Work out the finished part from the listing and answer in its coordinate system (mm). A direction names the side the tool comes from. Round coordinates to 2 decimals unless told otherwise and drop trailing zeros. Order: outer loops, then holes, each group sorted by start corner. A loop starts at its lowest first (then second) coordinate and runs counter-clockwise, first axis right, second up. Notation, with made-up numbers: (-33, -17) -> (21, -17) arc R20 cw to (21, 16) -> close; hole circle Ø3 at (-25, 83). An arc over 180 degrees is marked (long way). Use a Markdown table: item, result. Add a question column.
Item 1: For a pull along Z with two mould halves and no side action, classify faces 6 (the flat face through (90, 1, 0)), 7 (the flat face through (30.5, 5, 140)), 8 (the cylindrical face through (28.52, 3.48, 97.92)) as +Z half, -Z half, draft (parallel to the pull), parting line (faces both ways), or undercut.
Item 2: Flat-ended cylindrical pins translate along their axes: P1, Ø1, axis at x = 93, z = 76, coming from the -Y side; P2, Ø4, axis at x = 67.5, z = 99.5, coming from the +Y side; P3, Ø3, axis at x = 133, y = 5.5, coming from the +Z side. Find the tip coordinate at first contact, or state that the pin passes through.
Item 3: A cutting plane is placed at B-B, the plane z = 29. Determine the outline of the cut face in (x, y), plus the area to 3 significant figures.
Item 4: A cutting plane is placed at C-C, the plane y = -8. Determine the outline of the cut face in (x, z).
Item 5: A tool of negligible diameter and unlimited length cuts with its end or side. For faces 1 (the flat face through (71, 5, 13)), 2 (the flat face through (131, 7, 13)), 3 (the flat face through (144, 5, 90)), 4 (the flat face through (132, 5, 140)), 5 (the flat face through (81, 0, 77)), from which of +Z, -Z, +X, -X, +Y, -Y can it reach the whole face along a straight path? Write none if from no direction.
Item 6: Find the intervals of material crossed by L1, parallel to X at y = -2, z = 149; L2, parallel to Y at x = 5.5, z = 114.5; L3, parallel to Y at x = 178.5, z = 110.5, in increasing order. Write a range as [from, to].
Item 7: A cutting plane is placed at A-A, the plane z = 77.85. Determine the outline of the cut face in (x, y).
from build123d import *

# Parameters (mm, degrees)
LINEAR_AUSTRAGEN_D_NN1_DEPTH     = 155.5
SKIZZE7_R                        = 2.5
AUFSATZ_LINEAR_AUSTRAGEN3_DEPTH  = 5
SKIZZE8_R                        = 1.5
SCHNITT_LINEAR_AUSTRAGEN1_DEPTH  = 8
SKIZZE12_R                       = 1.5
SCHNITT_LINEAR_AUSTRAGEN4_DEPTH  = 8
SKIZZE13_R                       = 2.5
AUFSATZ_LINEAR_AUSTRAGEN5_DEPTH  = 5
SKIZZE16_R                       = 1.5
SCHNITT_LINEAR_AUSTRAGEN9_DEPTH  = 8
SKIZZE17_R                       = 1.5
SCHNITT_LINEAR_AUSTRAGEN10_DEPTH = 8
SKIZZE18_R                       = 2.5
AUFSATZ_LINEAR_AUSTRAGEN6_DEPTH  = 5
SKIZZE21_R                       = 1.5
SCHNITT_LINEAR_AUSTRAGEN13_DEPTH = 8
SKIZZE22_R                       = 1.5
SCHNITT_LINEAR_AUSTRAGEN14_DEPTH = 8
SKIZZE20_R                       = 1.2
AUFSATZ_LINEAR_AUSTRAGEN7_DEPTH  = 5
SKIZZE19_R                       = 1.2
AUFSATZ_LINEAR_AUSTRAGEN8_DEPTH  = 5
SKIZZE15_R                       = 1.2
AUFSATZ_LINEAR_AUSTRAGEN9_DEPTH  = 5
SKIZZE14_R                       = 1.2
AUFSATZ_LINEAR_AUSTRAGEN11_DEPTH = 5
SKIZZE10_R                       = 1.2
AUFSATZ_LINEAR_AUSTRAGEN12_DEPTH = 5
SKIZZE11_R                       = 1.2
AUFSATZ_LINEAR_AUSTRAGEN13_DEPTH = 5
CUT_EXTRUDE2_DEPTH               = 156.5
SKIZZE23_R                       = 13
SCHNITT_LINEAR_AUSTRAGEN15_DEPTH = 13
SKETCH5_W                        = 1
SKETCH5_H                        = 155.5
CUT_EXTRUDE_THIN1_DEPTH          = 1
SKETCH6_R                        = 2.5
SKETCH6_R_2                      = 1.5
BOSS_EXTRUDE1_DEPTH              = 5
CUT_EXTRUDE3_START               = -2
SKETCH7_R                        = 1.5
CUT_EXTRUDE3_DEPTH               = 2


with BuildPart() as part:
    # Skizze5 → Linear-Austragen-Dünn1 (new body)
    with BuildSketch(Plane.XY):
        with BuildLine():
            Line((-17.5, -12.340428851), (0, -12.340428851))
            Line((0, -12.340428851), (0, 0))
            Line((0, 0), (158.213118455, 0))
            Line((158.213118455, 0), (163.626964647, 0))
            ThreePointArc((163.626964647, 0), (171.029319744, 7.247508118), (181.129906705, 9.549545901))
            ThreePointArc((181.129906705, 9.549545901), (191.077251396, 6.131307404), (197.694328428, -2.044774322))
            Line((197.694328428, -2.044774322), (199.194328428, -2.044774322))
            Line((199.194328428, -2.044774322), (199.194328428, -0.044774322))
            Line((199.194328428, -0.044774322), (198.972575208, -0.044774322))
            ThreePointArc((198.972575208, -0.044774322), (191.667573532, 8.146277022), (181.232439294, 11.546915938))
            ThreePointArc((181.232439294, 11.546915938), (170.592452046, 9.278075868), (162.50625544, 2))
            Line((162.50625544, 2), (158.213118455, 2))
            Line((158.213118455, 2), (-2, 2))
            Line((-2, 2), (-2, -10.340428851))
            Line((-2, -10.340428851), (-17.5, -10.340428851))
            Line((-17.5, -10.340428851), (-17.5, -12.340428851))
        make_face()
    extrude(amount=LINEAR_AUSTRAGEN_D_NN1_DEPTH)

    # Skizze7 → Aufsatz-Linear austragen3 (add)
    with BuildSketch(Plane(origin=(0.013003032, 0, 0), x_dir=(1, 0, 0), z_dir=(0, 1, 0))):
        with Locations((11.5, -11.5)):
            Circle(SKIZZE7_R)
        with Locations((69.5, -11.5)):
            Circle(SKIZZE7_R)
        with Locations((11.5, -60.5)):
            Circle(SKIZZE7_R)
        with Locations((69.5, -60.5)):
            Circle(SKIZZE7_R)
    extrude(amount=AUFSATZ_LINEAR_AUSTRAGEN3_DEPTH)

    # Skizze8 → Schnitt-Linear austragen1 (cut)
    with BuildSketch(Plane(origin=(0, 5, 0), x_dir=(1, 0, 0), z_dir=(0, 1, 0))):
        with Locations((11.513003032, -11.5)):
            Circle(SKIZZE8_R)
    extrude(amount=-SCHNITT_LINEAR_AUSTRAGEN1_DEPTH, mode=Mode.SUBTRACT)

    # Skizze12 → Schnitt-Linear austragen4 (cut)
    with BuildSketch(Plane(origin=(0, 5, 0), x_dir=(1, 0, 0), z_dir=(0, 1, 0))):
        with Locations((69.513003032, -11.5)):
            Circle(SKIZZE12_R)
    extrude(amount=-SCHNITT_LINEAR_AUSTRAGEN4_DEPTH, mode=Mode.SUBTRACT)

    # Skizze13 → Aufsatz-Linear austragen5 (add)
    with BuildSketch(Plane(origin=(0.013003032, 0, 0), x_dir=(1, 0, 0), z_dir=(0, 1, 0))):
        with Locations((130, -140)):
            Circle(SKIZZE13_R)
        with Locations((102.1, -140)):
            Circle(SKIZZE13_R)
        with Locations((145.2, -89.2)):
            Circle(SKIZZE13_R)
        with Locations((97.4, -88.1)):
            Circle(SKIZZE13_R)
    extrude(amount=AUFSATZ_LINEAR_AUSTRAGEN5_DEPTH)

    # Skizze16 → Schnitt-Linear austragen9 (cut)
    with BuildSketch(Plane(origin=(0, 5, 0), x_dir=(1, 0, 0), z_dir=(0, 1, 0))):
        with Locations((102.113003032, -140)):
            Circle(SKIZZE16_R)
    extrude(amount=-SCHNITT_LINEAR_AUSTRAGEN9_DEPTH, mode=Mode.SUBTRACT)

    # Skizze17 → Schnitt-Linear austragen10 (cut)
    with BuildSketch(Plane(origin=(0, 5, 0), x_dir=(1, 0, 0), z_dir=(0, 1, 0))):
        with Locations((130.013003032, -140)):
            Circle(SKIZZE17_R)
    extrude(amount=-SCHNITT_LINEAR_AUSTRAGEN10_DEPTH, mode=Mode.SUBTRACT)

    # Skizze18 → Aufsatz-Linear austragen6 (add)
    with BuildSketch(Plane(origin=(0.013003032, 0, 0), x_dir=(1, 0, 0), z_dir=(0, 1, 0))):
        with Locations((68.430981836, -140)):
            Circle(SKIZZE18_R)
        with Locations((28.830981836, -140)):
            Circle(SKIZZE18_R)
        with Locations((28.83098184, -100.4)):
            Circle(SKIZZE18_R)
        with Locations((68.430981836, -100.4)):
            Circle(SKIZZE18_R)
    extrude(amount=AUFSATZ_LINEAR_AUSTRAGEN6_DEPTH)

    # Skizze21 → Schnitt-Linear austragen13 (cut)
    with BuildSketch(Plane(origin=(0, 5, 0), x_dir=(1, 0, 0), z_dir=(0, 1, 0))):
        with Locations((28.843984868, -140)):
            Circle(SKIZZE21_R)
    extrude(amount=-SCHNITT_LINEAR_AUSTRAGEN13_DEPTH, mode=Mode.SUBTRACT)

    # Skizze22 → Schnitt-Linear austragen14 (cut)
    with BuildSketch(Plane(origin=(0, 5, 0), x_dir=(1, 0, 0), z_dir=(0, 1, 0))):
        with Locations((68.443984868, -140)):
            Circle(SKIZZE22_R)
    extrude(amount=-SCHNITT_LINEAR_AUSTRAGEN14_DEPTH, mode=Mode.SUBTRACT)

    # Skizze20 → Aufsatz-Linear austragen7 (add)
    with BuildSketch(Plane(origin=(0, 5, 0), x_dir=(1, 0, 0), z_dir=(0, 1, 0))):
        with Locations((28.843984872, -100.4)):
            Circle(SKIZZE20_R)
    extrude(amount=AUFSATZ_LINEAR_AUSTRAGEN7_DEPTH)

    # Skizze19 → Aufsatz-Linear austragen8 (add)
    with BuildSketch(Plane(origin=(0, 5, 0), x_dir=(1, 0, 0), z_dir=(0, 1, 0))):
        with Locations((68.443984868, -100.4)):
            Circle(SKIZZE19_R)
    extrude(amount=AUFSATZ_LINEAR_AUSTRAGEN8_DEPTH)

    # Skizze15 → Aufsatz-Linear austragen9 (add)
    with BuildSketch(Plane(origin=(0, 5, 0), x_dir=(1, 0, 0), z_dir=(0, 1, 0))):
        with Locations((97.413003032, -88.1)):
            Circle(SKIZZE15_R)
    extrude(amount=AUFSATZ_LINEAR_AUSTRAGEN9_DEPTH)

    # Skizze14 → Aufsatz-Linear austragen11 (add)
    with BuildSketch(Plane(origin=(0, 5, 0), x_dir=(1, 0, 0), z_dir=(0, 1, 0))):
        with Locations((145.213003032, -89.2)):
            Circle(SKIZZE14_R)
    extrude(amount=AUFSATZ_LINEAR_AUSTRAGEN11_DEPTH)

    # Skizze10 → Aufsatz-Linear austragen12 (add)
    with BuildSketch(Plane(origin=(0, 5, 0), x_dir=(1, 0, 0), z_dir=(0, 1, 0))):
        with Locations((11.513003032, -60.5)):
            Circle(SKIZZE10_R)
    extrude(amount=AUFSATZ_LINEAR_AUSTRAGEN12_DEPTH)

    # Skizze11 → Aufsatz-Linear austragen13 (add)
    with BuildSketch(Plane(origin=(0, 5, 0), x_dir=(1, 0, 0), z_dir=(0, 1, 0))):
        with Locations((69.513003032, -60.5)):
            Circle(SKIZZE11_R)
    extrude(amount=AUFSATZ_LINEAR_AUSTRAGEN13_DEPTH)

    # Sketch3 → Cut-Extrude2 (cut, through all)
    with BuildSketch(Plane(origin=(0, 0, 0), x_dir=(-1, 0, 0), z_dir=(0, 0, -1))):
        Polygon((17.5, -10.340428851), (15.5, -12.340428851), (17.5, -12.340428851), align=None)
    extrude(amount=-CUT_EXTRUDE2_DEPTH, mode=Mode.SUBTRACT)

    # Skizze23 → Schnitt-Linear austragen15 (cut)
    with BuildSketch(Plane(origin=(0, 2, 0), x_dir=(1, 0, 0), z_dir=(0, 1, 0))):
        with Locations((181, -77.85)):
            Circle(SKIZZE23_R)
    extrude(amount=SCHNITT_LINEAR_AUSTRAGEN15_DEPTH, mode=Mode.SUBTRACT)

    # Sketch5 → Cut-Extrude-Thin1 (cut)
    with BuildSketch(Plane(origin=(0, 2, 0), x_dir=(1, 0, 0), z_dir=(0, 1, 0))):
        with Locations((80.25312772, -77.75)):
            Rectangle(SKETCH5_W, SKETCH5_H)
    extrude(amount=-CUT_EXTRUDE_THIN1_DEPTH, mode=Mode.SUBTRACT)

    # Sketch6 → Boss-Extrude1 (add)
    with BuildSketch(Plane(origin=(0, 2, 0), x_dir=(1, 0, 0), z_dir=(0, 1, 0))):
        with Locations((130.01300303, -11.5)):
            Circle(SKETCH6_R)
        with Locations((130.01300303, -11.5)):
            Circle(SKETCH6_R_2, mode=Mode.SUBTRACT)
    extrude(amount=BOSS_EXTRUDE1_DEPTH)

    # Sketch7 → Cut-Extrude3 (cut)
    with BuildSketch(Plane(origin=(0, 2, 0), x_dir=(1, 0, 0), z_dir=(0, 1, 0)).offset(CUT_EXTRUDE3_START)):
        with Locations((130.01300303, -11.5)):
            Circle(SKETCH7_R)
    extrude(amount=CUT_EXTRUDE3_DEPTH, mode=Mode.SUBTRACT)


solid = part.part
Reported:
| question | item | result |
|---|---|---|
| 1 | face 6 | -Z half |
| 1 | face 7 | draft |
| 1 | face 8 | undercut |
| 2 | P1 | y = 0 |
| 2 | P2 | y = 10 |
| 2 | P3 | z = 141.94 |
| 3 | outline | (-17.5, -10.34) -> (-15.5, -12.34) -> (0, -12.34) -> (0, 0) -> (163.63, 0) arc R19.05 cw to (197.69, -2.04) -> (199.19, -2.04) -> (199.19, -0.04) -> (198.97, -0.04) arc R21.05 ccw to (162.51, 2) -> (80.75, 2) -> (80.75, 1) -> (79.75, 1) -> (79.75, 2) -> (-2, 2) -> (-2, -10.34) -> close |
| 3 | area | 471 mm² |
| 4 | outline | (-2, 0) -> (0, 0) -> (0, 155.5) -> (-2, 155.5) -> close |
| 5 | face 1 | -Z, -X, +Y |
| 5 | face 2 | +Z, -Z, -X, +Y |
| 5 | face 3 | +Y |
| 5 | face 4 | +Z, -X, +Y |
| 5 | face 5 | +Z, -Z, -Y |
| 6 | L1 | [-2, 0], [197.68, 199.19] |
| 6 | L2 | [0, 2] |
| 6 | L3 | [9.5, 11.51] |
| 7 | outline | (-17.5, -10.34) -> (-15.5, -12.34) -> (0, -12.34) -> (0, 0) -> (163.63, 0) arc R19.05 cw to (168, 5.19) -> (168, 7.71) arc R21.05 ccw to (162.51, 2) -> (80.75, 2) -> (80.75, 1) -> (79.75, 1) -> (79.75, 2) -> (-2, 2) -> (-2, -10.34) -> close; (194, 3.61) arc R19.05 cw to (197.69, -2.04) -> (199.19, -2.04) -> (199.19, -0.04) -> (198.97, -0.04) arc R21.05 ccw to (194, 6.38) -> close |
